```python
from build123d import *

# Parameters (mm, degrees)
SKETCH009_R           = 3.5
PAD006_DEPTH          = 0.5
CHAMFER001_SIZE       = 0.25
SKETCH010_R           = 3
PAD007_DEPTH          = 8
CHAMFER002_SIZE       = 0.5
POCKET002_DEPTH       = 6.5
POLARPATTERN002_COUNT = 18
SKETCH012_W           = 6.5
SKETCH012_H           = 1
POCKET003_DEPTH       = 6.5


with BuildPart() as part:
    # Sketch009 → Pad006 (new body)
    with BuildSketch(Plane.XY.offset(18.5)):
        Circle(SKETCH009_R)
    extrude(amount=PAD006_DEPTH)

    # Chamfer001
    chamfer001_edges = [part.edges().sort_by_distance(p)[0] for p in [
        (-3.5, 0, 19),
    ]]
    chamfer(chamfer001_edges, length=CHAMFER001_SIZE)

    # Sketch010 (on Face4 of Chamfer001) → Pad007 (join)
    with BuildSketch(Plane.XY.offset(19)):
        Circle(SKETCH010_R)
    extrude(amount=PAD007_DEPTH)

    # Chamfer002
    chamfer002_edges = [part.edges().sort_by_distance(p)[0] for p in [
        (-3, 0, 27),
    ]]
    chamfer(chamfer002_edges, length=CHAMFER002_SIZE)

    # Sketch011 (on Face6 of Pad007) → Pocket002 (cut)
    with BuildSketch(Plane.XY.offset(27)):
        Polygon((0, 2.5), (0.433013, 3.25), (-0.433013, 3.25), align=None)
    pocket002 = extrude(amount=-POCKET002_DEPTH, mode=Mode.SUBTRACT)

    # PolarPattern002: Pocket002 ×18 about axis
    polarpattern002_axis = Axis((0, 0, 27), (0, 0, 1))
    for i in range(1, POLARPATTERN002_COUNT):
        add(pocket002.rotate(polarpattern002_axis, i * 360 / POLARPATTERN002_COUNT), mode=Mode.SUBTRACT)

    # Sketch012 (on Face76 of PolarPattern002) → Pocket003 (cut)
    with BuildSketch(Plane.XY.offset(27)):
        Rectangle(SKETCH012_W, SKETCH012_H)
    extrude(amount=-POCKET003_DEPTH, mode=Mode.SUBTRACT)


solid = part.part
```
Source: CAD feature listing. Evaluate the final solid. Frame: model axes, mm. A direction names the side the tool comes from. Coordinates: 2 decimals unless noted, no trailing zeros. Loops run counter-clockwise (first coordinate to the right, second up) from the corner with the lowest first, then second, coordinate; pieces in that order, holes last. Notation, with made-up numbers: M 62,77 L 88,77 A9 cw 88,87 Z; hole C 89,73.5 d10. An arc over 180 degrees is marked long. Use CSV: the item, a comma, the result in double quotes.
(1) Cut plane B-B on z = 20. Return loops of the section in (x, y).
Answers follow:
outline,"C 0,0 d6"
(2) Reachability of faces 1 (the face through (0, 1, 27)), 2 (the face through (0, -0.5, 24)) from +Z, -Z, +X, -X, +Y, -Y: full face, straight path, thin tool, end or side. Return the list, or none.
Answers follow:
face 1,"+Z, +X, -X, +Y, -Y"
face 2,"+Z, +X, -X"
(3) Draft query along Y for faces 3 (the face through (0, 0, 20.5)), 4 (the face through (2.1, 1.7, 26.8)), 5 (the face through (0, 0, 18.5)). Return one class per face: pulls with the +Y half, pulls with the -Y half, needs draft (parallel to the pull), parting line crosses it, or undercut.
Answers follow:
face 3,"undercut"
face 4,"pulls with the +Y half"
face 5,"needs draft"
(4) Line query: line 1 (Y direction, x = -1, z = 24.5); line 2 (X direction, y = 0.25, z = 20); line 3 (Y direction, x = 0.5, z = 22.5). Output: solid intervals per line, ascending. Write a range as [from, to].
Answers follow:
line 1,"[-2.47, -0.5], [0.5, 2.47]"
line 2,"[-2.99, 2.99]"
line 3,"[-2.96, -0.5], [0.5, 2.96]"
(5) Cut plane A-A on y = 0. Return loops of the section in (x, z).
Answers follow:
outline,"M -3.5,18.5 L 3.5,18.5 L 3.5,18.75 L 3.25,19 L 3,19 L 3,20.5 L -3,20.5 L -3,19 L -3.25,19 L -3.5,18.75 Z"
(6) Contact query for flat-ended pins moving along their axis: pin 1 (3 mm diameter, centred on y = 1.5, z = 24.5, fed in from +X); pin 2 (0.6 mm diameter, centred on x = 2.5, z = 25, fed in from +Y); pin 3 (0.6 mm diameter, centred on x = -2.5, z = 25.5, fed in from -Y); pin 4 (0.6 mm diameter, centred on x = -1, y = -2.5, fed in from +Z). Output: stop coordinate, or through.
Answers follow:
pin 1,"x = 2.89"
pin 2,"y = 2.04"
pin 3,"y = -2.04"
pin 4,"z = 27"
